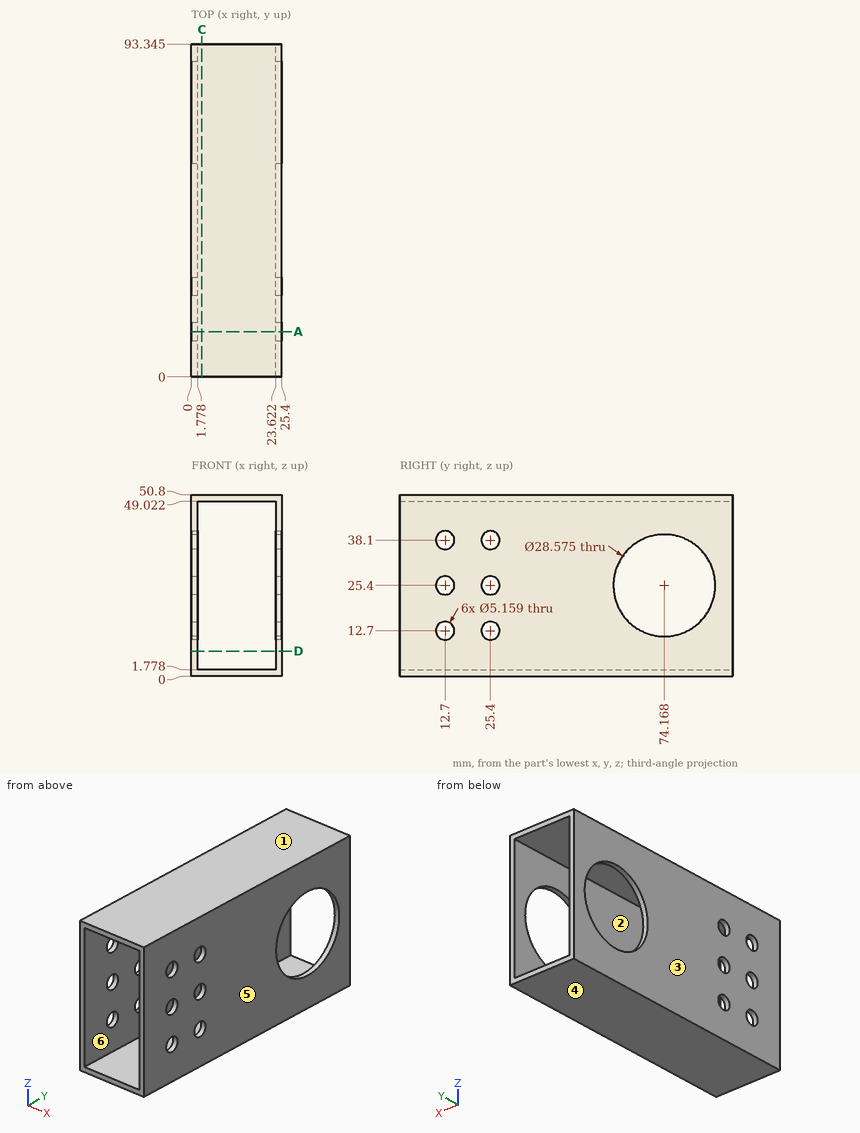
Job drawing, mm, ordinate dimensions from the low corner. One solid piece. A direction names the side the tool comes from. Round coordinates to 2 decimals unless told otherwise and drop trailing zeros. Order: outer loops, then holes, each group sorted by start corner. A loop starts at its lowest first (then second) coordinate and runs counter-clockwise, first axis right, second up. Notation, with made-up numbers: (76, -28) -> (85, -28) arc R32 cw to (85, 5) -> close; hole circle Ø2 at (57.5, 17.5). An arc over 180 degrees is marked (long way). Answer in a Markdown table with one row per item.
1) Band-saw the part on D-D on z = 7. Give the cut face in (x, y) (1 decimal), and give its area (3 significant figures).
Values:
| item | result |
|---|---|
| outline | (0, 0) -> (1.8, 0) -> (1.8, 93.3) -> (0, 93.3) -> close; (23.6, 0) -> (25.4, 0) -> (25.4, 93.3) -> (23.6, 93.3) -> close |
| area | 332 mm2 |
2) Mould opens along X. For the marked faces 3, 4, 5 and 6 say: released by +X, released by -X, zero draft, split by the parting line, or undercut.
Values:
| item | result |
|---|---|
| face 3 | released by -X |
| face 4 | zero draft |
| face 5 | released by +X |
| face 6 | undercut |
3) Which spindle directions (+Z, -Z, +X, -X, +Y, -Y) get a long thin tool onto all of the face, cutting with end or side? Do the marked faces 1 and 2. Say none if no direction does.
Values:
| item | result |
|---|---|
| face 1 | +Z, +X, -X, +Y, -Y |
| face 2 | +Y, -Y |
4) Band-saw the part on C-C on x = 3. Give the cut face in (y, z) (1 decimal).
Values:
| item | result |
|---|---|
| outline | (0, 0) -> (93.3, 0) -> (93.3, 1.8) -> (0, 1.8) -> close; (0, 49) -> (93.3, 49) -> (93.3, 50.8) -> (0, 50.8) -> close |
5) Wall check: L1, parallel to Y at x = 24.6, z = 25.4 (1 decimal); L2, parallel to Z at x = 5.75, y = 46; L3, parallel to X at y = 30, z = 29.5. Give the ranges that are in metal, low to high.
Values:
| item | result |
|---|---|
| L1 | 0 to 10.1, 15.3 to 22.8, 28 to 59.9, 88.5 to 93.3 |
| L2 | 0 to 1.78, 49.02 to 50.8 |
| L3 | 0 to 1.78, 23.62 to 25.4 |
6) Band-saw the part on A-A on y = 12.7. Give the number of separate pieces and of enclosed holes in the cut face, and give its area (3 significant figures).
Values:
| item | result |
|---|---|
| separate pieces | 6 |
| enclosed holes | 0 |
| area | 203 mm2 |
